Verification items for the finished model (mm, model axes). A direction names the side the tool comes from. Round coordinates to 2 decimals unless told otherwise and drop trailing zeros. Write each loop counter-clockwise with the first axis right and the second up, starting at its lowest first coordinate (ties: lowest second). Pieces come first, ordered by that corner, then holes.
from build123d import *

# Parameters (mm, degrees)
PAD_DEPTH       = 2
SKETCH007_W     = 10
SKETCH007_H     = 60
SKETCH007_W_2   = 59.5
SKETCH007_H_2   = 40
POCKET001_DEPTH = 2
SKETCH016_W     = 10
SKETCH016_H     = 20
PAD006_DEPTH    = 10
SKETCH014_R     = 1.5
POCKET002_DEPTH = 2
SKETCH015_R     = 1.5
POCKET003_DEPTH = 2
SKETCH036_W     = 10
SKETCH036_H     = 20
PAD018_DEPTH    = 10
SKETCH037_R     = 1.5
POCKET009_DEPTH = 2
SKETCH038_R     = 1.5
POCKET010_DEPTH = 2
SKETCH059_W     = 60
SKETCH059_H     = 2
PAD033_DEPTH    = 4.25
SKETCH063_W     = 20
SKETCH063_H     = 20
PAD037_DEPTH    = 10
SKETCH065_W     = 10
SKETCH065_H     = 20
PAD038_DEPTH    = 22
SKETCH066_W     = 20
SKETCH066_H     = 20
PAD039_DEPTH    = 10


with BuildPart() as part:
    # Sketch → Pad (new body)
    with BuildSketch(Plane.XY):
        Polygon((0, 0), (0, 190), (10, 200), (95, 200), (105, 190), (105, 0), align=None)
    extrude(amount=PAD_DEPTH)

    # Sketch007 (on Face8 of Pad) → Pocket001 (cut)
    with BuildSketch(Plane.XY.offset(2)):
        with Locations((5, 50)):
            Rectangle(SKETCH007_W, SKETCH007_H)
        with Locations((100, 50)):
            Rectangle(SKETCH007_W, SKETCH007_H)
        with Locations((5, 145)):
            Rectangle(SKETCH007_W, SKETCH007_H)
        with Locations((100, 145)):
            Rectangle(SKETCH007_W, SKETCH007_H)
        with Locations((52.5, 52)):
            Rectangle(SKETCH007_W_2, SKETCH007_H_2)
    extrude(amount=-POCKET001_DEPTH, mode=Mode.SUBTRACT)

    # Sketch016 → Pad006 (join)
    with BuildSketch(Plane.XZ.offset(-45)):
        with Locations((15, 12)):
            Rectangle(SKETCH016_W, SKETCH016_H)
        with Locations((90, 12)):
            Rectangle(SKETCH016_W, SKETCH016_H)
    extrude(amount=-PAD006_DEPTH)

    # Sketch014 → Pocket002 (cut)
    with BuildSketch(Plane.YZ.offset(10)):
        with Locations((50, 14)):
            Circle(SKETCH014_R)
    extrude(amount=POCKET002_DEPTH, mode=Mode.SUBTRACT)

    # Sketch015 → Pocket003 (cut)
    with BuildSketch(Plane.YZ.offset(95)):
        with Locations((50, 14)):
            Circle(SKETCH015_R)
    extrude(amount=-POCKET003_DEPTH, mode=Mode.SUBTRACT)

    # Sketch036 → Pad018 (join)
    with BuildSketch(Plane.XZ.offset(-140)):
        with Locations((90, 12)):
            Rectangle(SKETCH036_W, SKETCH036_H)
        with Locations((15, 12)):
            Rectangle(SKETCH036_W, SKETCH036_H)
    extrude(amount=-PAD018_DEPTH)

    # Sketch037 (on Face42 of Pad018) → Pocket009 (cut)
    with BuildSketch(Plane(origin=(10, 0, 0), x_dir=(0, -1, 0), z_dir=(-1, 0, 0))):
        with Locations((-145, 14)):
            Circle(SKETCH037_R)
    extrude(amount=-POCKET009_DEPTH, mode=Mode.SUBTRACT)

    # Sketch038 (on Face43 of Pad018) → Pocket010 (cut)
    with BuildSketch(Plane.YZ.offset(95)):
        with Locations((145, 14)):
            Circle(SKETCH038_R)
    extrude(amount=-POCKET010_DEPTH, mode=Mode.SUBTRACT)

    # Sketch059 (on Face4 of Pocket010) → Pad033 (join)
    with BuildSketch(Plane.XY.offset(2)):
        with Locations((52.5, 157.48)):
            Rectangle(SKETCH059_W, SKETCH059_H)
        with Locations((52.5, 149.68)):
            Rectangle(SKETCH059_W, SKETCH059_H)
    extrude(amount=PAD033_DEPTH)

    # Sketch063 (on Face35 of Pad033) → Pad037 (join)
    with BuildSketch(Plane.XZ.offset(-140)):
        with Locations((20, 12)):
            Rectangle(SKETCH063_W, SKETCH063_H)
        with Locations((85, 12)):
            Rectangle(SKETCH063_W, SKETCH063_H)
    extrude(amount=PAD037_DEPTH)

    # Sketch065 (on Face29 of Pad037) → Pad038 (join)
    with BuildSketch(Plane.XZ.offset(-45)):
        with Locations((15, 12)):
            Rectangle(SKETCH065_W, SKETCH065_H)
        with Locations((90, 12)):
            Rectangle(SKETCH065_W, SKETCH065_H)
    extrude(amount=PAD038_DEPTH)

    # Sketch066 (on Face29 of Pad038) → Pad039 (join)
    with BuildSketch(Plane.XZ.offset(-23)):
        with Locations((20, 12)):
            Rectangle(SKETCH066_W, SKETCH066_H)
        with Locations((85, 12)):
            Rectangle(SKETCH066_W, SKETCH066_H)
    extrude(amount=PAD039_DEPTH)


solid = part.part
Q1. Release check for a two-part mould opening along Y. For faces 6 (the flat face through (100, 195, 1)), 7 (the flat face through (30, 18, 12)), 8 (the flat face through (85, 13, 12)), 9 (the flat face through (53, 101, 2)) record: released by +Y, released by -Y, zero draft, split by the parting line, or undercut.
Recorded:
face 6: released by +Y
face 7: zero draft
face 8: released by -Y
face 9: undercut
Q2. Tool access check on faces 1 (the flat face through (25, 23, 12)), 2 (the flat face through (75, 18, 12)), 3 (the flat face through (90, 150, 12)), 4 (the flat face through (85, 130, 12)), 5 (the flat face through (20, 13, 12)). Record the directions out of +Z, -Z, +X, -X, +Y, -Y that give a thin tool (end or side, any length) a straight path to the whole face; none if there is none.
Recorded:
face 1: +Z
face 2: +Z, -Y
face 3: +Z, +X, +Y
face 4: +Z, +X, -X
face 5: +Z, +X, -X, -Y
Q3. Sectioned sample at A-A (z = 8.75). Enter the section's corners in (x, y).
Recorded:
outline: (10, 13) - (30, 13) - (30, 23) - (20, 23) - (20, 55) - (10, 55) - close; (10, 130) - (30, 130) - (30, 140) - (20, 140) - (20, 150) - (10, 150) - close; (75, 13) - (95, 13) - (95, 55) - (85, 55) - (85, 23) - (75, 23) - close; (75, 130) - (95, 130) - (95, 150) - (85, 150) - (85, 140) - (75, 140) - close
Q4. Material ranges on line 1 along Y through (x, z) = (78, 7); line 2 along Z through (x, y) = (11.15, 50); line 3 along Y through (x, z) = (89.5, 15.5), recorded low to high.
Recorded:
line 1: y = 13 to 23, 130 to 140
line 2: z = 0 to 12.5, 15.5 to 22
line 3: y = 13 to 55, 130 to 150
Q5. Sectioned sample at C-C (y = 43). Enter the section's corners in (x, z), plus the area to 3 significant figures.
Recorded:
outline: (10, 0) - (22.75, 0) - (22.75, 2) - (20, 2) - (20, 22) - (10, 22) - close; (82.25, 0) - (95, 0) - (95, 22) - (85, 22) - (85, 2) - (82.25, 2) - close
area: 451 mm2
Q6. Depth check by flat-ended pin: P1, Ø0.9, axis at y = 144.5, z = 14.5, coming from the -X side; P2, Ø8, axis at x = 15, z = 12, coming from the +Y side; P3, Ø1.6, axis at y = 149.5, z = 3.5, coming from the -X side. Enter the tip coordinate at first touch or a pass-through.
Recorded:
P1: stops at x = 12
P2: stops at y = 150
P3: stops at x = 10
Q7. Sectioned sample at B-B (x = 67). Enter the section's corners in (y, z), plus the area to 3 significant figures.
Recorded:
outline: (0, 0) - (32, 0) - (32, 2) - (0, 2) - close; (72, 0) - (200, 0) - (200, 2) - (158.48, 2) - (158.48, 6.25) - (156.48, 6.25) - (156.48, 2) - (150.68, 2) - (150.68, 6.25) - (148.68, 6.25) - (148.68, 2) - (72, 2) - close
area: 337 mm2
